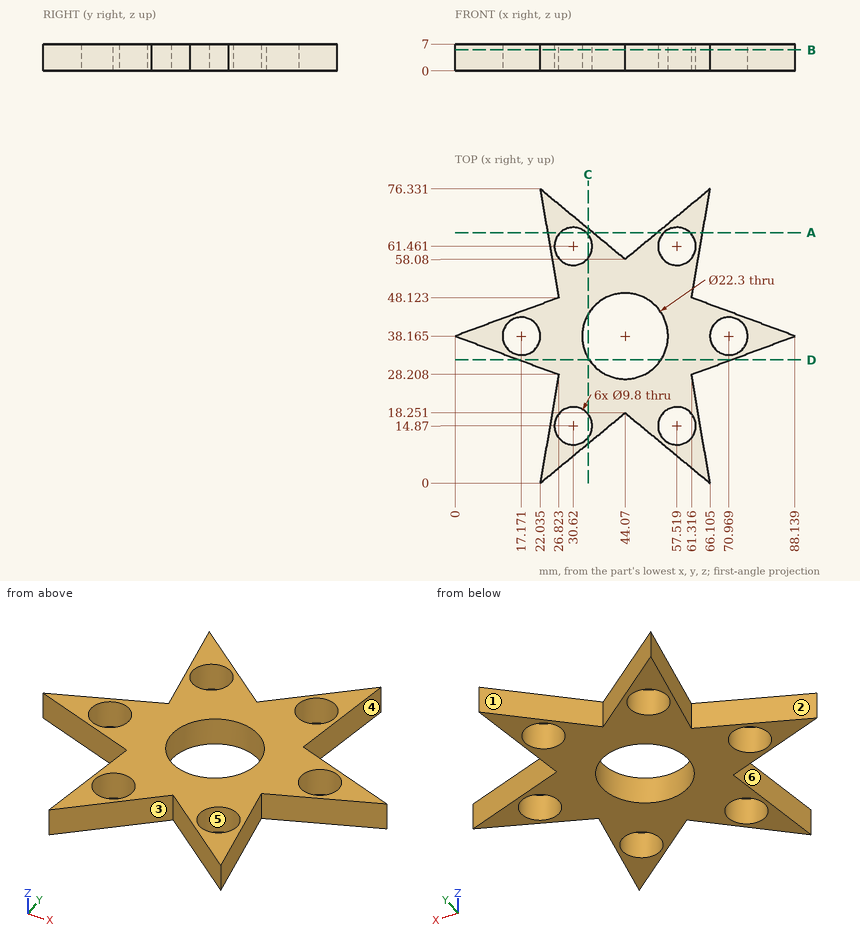
Could you check a few things on this drawing? It's one solid part, dimensions in mm from its lowest x, y, z. A direction names the side the tool comes from. Coordinates: 2 decimals unless noted, no trailing zeros. Loops run counter-clockwise (first coordinate to the right, second up) from the corner with the lowest first, then second, coordinate; pieces in that order, holes last. Notation, with made-up numbers: (-25.5, -37.5) - (-1.5, -37.5) arc R26 cw to (-1.5, -0.5) - close; hole circle Ø1 at (-3, -30.75). An arc over 180 degrees is marked (long way). Answer as a JSON object with one key per item and string values. Group by question number.
Item 1: If we mould it in two halves opening along Y, with no side actions, what happens to the marked faces 1, 2 and 3? For each: released by +Y, released by -Y, zero draft, split by the parting line, or undercut.
Item 2: If we section it at A-A (y = 65): List the corners of the cut face in (x, z) for me (1 decimal).
Item 3: If we section it at C-C (x = 34.5): List the corners of the cut face in (y, z) for me (1 decimal), plus the area to 3 significant figures.
Item 4: On a 3-axis mill with a long thin cutter (end or side, diameter ignored), from which of +Z, -Z, +X, -X, +Y, -Y can I reach the whole of each face in a straight line? I mean the marked faces 4, 5 and 6. Say none if no direction works.
Item 5: If we section it at B-B (z = 5.5): State how many separate pieces and enclosed holes the cut face has, plus the area to 3 significant figures.
Item 6: If we section it at D-D (y = 32): List the corners of the cut face in (x, z) for me.
Item 7: For pin 1 (12.5 mm diameter, centred on x = 70.97, y = 38.17, fed in from +Z); pin 2 (1.5 mm diameter, centred on x = 44, z = 4, fed in from -Y); pin 3 (8 mm diameter, centred on x = 17.17, y = 38.17, fed in from -Z); pin 4 (1.5 mm diameter, centred on y = 38.5, z = 3.5, fed in from -X), each with a flat end and sliding along its axis, tell me the tip position at first contact or that it passes through.
Item 8: If I drill on L1, parallel to Y at x = 61, z = 5.75 (1 decimal); L2, parallel to X at y = 59, z = 2.25 (1 decimal); L3, parallel to X at y = 17, z = 2.5 (1 decimal), over which ranges is the centre line in solid material (lowest first)? Write a range as from..to.
Returned:
{
 "1": {"face 1": "released by +Y", "face 2": "undercut", "face 3": "released by -Y"},
 "2": {"outline": "(24, 0) - (27.2, 0) - (27.2, 7) - (24, 7) - close; (34, 0) - (35.7, 0) - (35.7, 7) - (34, 7) - close; (52.4, 0) - (54.1, 0) - (54.1, 7) - (52.4, 7) - close; (60.9, 0) - (64.2, 0) - (64.2, 7) - (60.9, 7) - close"},
 "3": {"outline": "(10.3, 0) - (11.9, 0) - (11.9, 7) - (10.3, 7) - close; (17.9, 0) - (32.4, 0) - (32.4, 7) - (17.9, 7) - close; (43.9, 0) - (58.5, 0) - (58.5, 7) - (43.9, 7) - close; (64.5, 0) - (66, 0) - (66, 7) - (64.5, 7) - close", "area": "226 mm²"},
 "4": {"face 4": "+Z, -Z, +X", "face 5": "+Z, -Z", "face 6": "+Z, -Z, -X"},
 "5": {"separate pieces": "1", "enclosed holes": "7", "area": "1,790 mm²"},
 "6": {"outline": "(16.61, 0) - (34.78, 0) - (34.78, 7) - (16.61, 7) - close; (53.36, 0) - (71.53, 0) - (71.53, 7) - (53.36, 7) - close"},
 "7": {"pin 1": "stops at z = 7", "pin 2": "stops at y = 17.57", "pin 3": "passes through", "pin 4": "stops at x = 0"},
 "8": {"L1": "y = 4.2..11.4, 18.3..58, 64.9..72.1", "L2": "x = 25..26.4, 34.9..43, 45.2..53.3, 61.8..63.2", "L3": "x = 24.9..26.2, 35..42.6, 45.6..53.1, 61.9..63.2"}
}
